The listing builds one solid part. Answer for the finished solid, in the listing's coordinates (mm). A direction names the side the tool comes from. Coordinates: 2 decimals unless noted, no trailing zeros. Write each loop counter-clockwise with the first axis right and the second up, starting at its lowest first coordinate (ties: lowest second). Pieces come first, ordered by that corner, then holes.
```python
from build123d import *

# Parameters (mm, degrees)
SKETCH1_W           = 30.5
SKETCH1_H           = 15
BOSS_EXTRUDE1_DEPTH = 60
SKETCH2_R           = 4.1
CUT_EXTRUDE1_DEPTH  = 16
SKETCH3_R           = 1.6
CUT_EXTRUDE2_DEPTH  = 15


with BuildPart() as part:
    # Sketch1 → Boss-Extrude1 (new body)
    with BuildSketch(Plane(origin=(0, 0, 0), x_dir=(1, 0, 0), z_dir=(0, 1, 0))):
        Rectangle(SKETCH1_W, SKETCH1_H)
    extrude(amount=BOSS_EXTRUDE1_DEPTH)

    # Sketch2 → Cut-Extrude1 (cut, through all)
    with BuildSketch(Plane.XY.offset(7.5)):
        with Locations((-6.25, 51)):
            Circle(SKETCH2_R)
        with Locations((-6.25, 9)):
            Circle(SKETCH2_R)
    extrude(amount=-CUT_EXTRUDE1_DEPTH, mode=Mode.SUBTRACT)

    # Sketch3 → Cut-Extrude2 (cut)
    with BuildSketch(Plane(origin=(15.25, 0, 0), x_dir=(0, 0, -1), z_dir=(1, 0, 0))):
        with Locations((0, 51)):
            Circle(SKETCH3_R)
        with Locations((0, 9)):
            Circle(SKETCH3_R)
    extrude(amount=-CUT_EXTRUDE2_DEPTH, mode=Mode.SUBTRACT)


solid = part.part
```
(1) This flat-tipped pin is pushed along its axis until it touches: pin 1 (1.9 mm diameter, centred on y = 51, z = 0, fed in from +X). Where does it stop, or does it pass through?
(2) Section B-B, the plane x = -6.25 is taken. Write down the section's boundary in (y, z).
(3) Which of the six approach directions +Z, -Z, +X, -X, +Y, -Y give full straight-line access (tool end or side, diameter ignored) to faces 4 (the cylindrical face through (-4.05, 54.46, 0.11)), 5 (the cylindrical face through (7.86, 52.35, -0.86))?
(4) Section D-D, the plane x = 6.5 is taken. Write down the section's boundary in (y, z).
(5) For a pull along Y with two mould halves and no side action, classify faces 1 (the flat face through (0, 0, 0)), 2 (the flat face through (15.25, 30, 0)), 3 (the cylindrical face through (7.86, 7.44, 0.35)) as pulls with the +Y half, pulls with the -Y half, needs draft (parallel to the pull), parting line crosses it, or undercut.
(6) Section C-C, the plane z = 0 is taken. Write down the section's boundary in (x, y), plus the area to 3 significant figures.
(7) Find the intervals of material crossed by probe 1 along Y at (x, z) = (11.75, 0); probe 2 along Y at (x, z) = (-6.25, -4); probe 3 along Z at (x, y) = (13.5, 50.5), in increasing order.
(8) Section A-A, the plane y = 9 is taken. Write down the section's boundary in (x, z).
Solution:
1. pin 1: stops at x = 0.25
2. outline: (0, -7.5) - (4.9, -7.5) - (4.9, 7.5) - (0, 7.5) - close; (13.1, -7.5) - (46.9, -7.5) - (46.9, 7.5) - (13.1, 7.5) - close; (55.1, -7.5) - (60, -7.5) - (60, 7.5) - (55.1, 7.5) - close
3. face 4: +Z, -Z
3. face 5: +X
4. outline: (0, -7.5) - (60, -7.5) - (60, 7.5) - (0, 7.5) - close; hole circle Ø3.2 at (9, 0); hole circle Ø3.2 at (51, 0)
5. face 1: pulls with the -Y half
5. face 2: needs draft
5. face 3: undercut
6. outline: (-15.25, 0) - (15.25, 0) - (15.25, 7.4) - (0.25, 7.4) - (0.25, 10.6) - (15.25, 10.6) - (15.25, 49.4) - (0.25, 49.4) - (0.25, 52.6) - (15.25, 52.6) - (15.25, 60) - (-15.25, 60) - close; hole circle Ø8.2 at (-6.25, 9); hole circle Ø8.2 at (-6.25, 51)
6. area: 1,630 mm2
7. probe 1: y = 0 to 7.4, 10.6 to 49.4, 52.6 to 60
7. probe 2: y = 0 to 4.9, 13.1 to 46.9, 55.1 to 60
7. probe 3: z = -7.5 to -1.52, 1.52 to 7.5
8. outline: (-15.25, -7.5) - (-10.35, -7.5) - (-10.35, 7.5) - (-15.25, 7.5) - close; (-2.15, -7.5) - (15.25, -7.5) - (15.25, -1.6) - (0.25, -1.6) - (0.25, 1.6) - (15.25, 1.6) - (15.25, 7.5) - (-2.15, 7.5) - close
